```python
from build123d import *

# Parameters (mm, degrees)
SKETCH8_W           = 114.3
SKETCH8_H           = 38.1
BOSS_EXTRUDE3_DEPTH = 19.05


with BuildPart() as part:
    # Sketch8 → Boss-Extrude3 (new body)
    with BuildSketch(Plane.XY):
        with BuildLine():
            Line((-257.351483657, 282.913503235), (-304.976483657, 282.913503235))
            Line((-304.976483657, 282.913503235), (-304.976483657, 244.813503235))
            ThreePointArc((-304.976483657, 244.813503235), (-301.801483657, 241.638503235), (-304.976483657, 238.463503235))
            Line((-304.976483657, 238.463503235), (-324.026483657, 238.463503235))
            Line((-324.026483657, 238.463503235), (-324.026483657, 219.413503235))
            Line((-324.026483657, 219.413503235), (-304.976483657, 219.413503235))
            ThreePointArc((-304.976483657, 219.413503235), (-301.801483657, 216.238503235), (-304.976483657, 213.063503235))
            Line((-304.976483657, 213.063503235), (-304.976483657, 111.463503235))
            ThreePointArc((-304.976483657, 111.463503235), (-301.801483657, 108.288503235), (-304.976483657, 105.113503235))
            Line((-304.976483657, 105.113503235), (-324.026483657, 105.113503235))
            Line((-324.026483657, 105.113503235), (-324.026483657, 86.063503235))
            Line((-324.026483657, 86.063503235), (-304.976483657, 86.063503235))
            ThreePointArc((-304.976483657, 86.063503235), (-301.801483657, 82.888503235), (-304.976483657, 79.713503235))
            Line((-304.976483657, 79.713503235), (-304.976483657, -21.886496765))
            ThreePointArc((-304.976483657, -21.886496765), (-301.801483657, -25.061496765), (-304.976483657, -28.236496765))
            Line((-304.976483657, -28.236496765), (-324.026483657, -28.236496765))
            Line((-324.026483657, -28.236496765), (-324.026483657, -47.286496765))
            Line((-324.026483657, -47.286496765), (-304.976483657, -47.286496765))
            ThreePointArc((-304.976483657, -47.286496765), (-301.801483657, -50.461496765), (-304.976483657, -53.636496765))
            Line((-304.976483657, -53.636496765), (-304.976483657, -155.236496765))
            ThreePointArc((-304.976483657, -155.236496765), (-301.801483657, -158.411496765), (-304.976483657, -161.586496765))
            Line((-304.976483657, -161.586496765), (-324.026483657, -161.586496765))
            Line((-324.026483657, -161.586496765), (-324.026483657, -180.636496765))
            Line((-324.026483657, -180.636496765), (-304.976483657, -180.636496765))
            ThreePointArc((-304.976483657, -180.636496765), (-301.801483657, -183.811496765), (-304.976483657, -186.986496765))
            Line((-304.976483657, -186.986496765), (-304.976483657, -266.361496765))
            Line((-304.976483657, -266.361496765), (304.623516343, -266.361496765))
            Line((304.623516343, -266.361496765), (304.623516343, -186.986496765))
            ThreePointArc((304.623516343, -186.986496765), (301.448516343, -183.811496765), (304.623516343, -180.636496765))
            Line((304.623516343, -180.636496765), (323.673516343, -180.636496765))
            Line((323.673516343, -180.636496765), (323.673516343, -161.586496765))
            Line((323.673516343, -161.586496765), (304.623516343, -161.586496765))
            ThreePointArc((304.623516343, -161.586496765), (301.448516343, -158.411496765), (304.623516343, -155.236496765))
            Line((304.623516343, -155.236496765), (304.623516343, -53.636496765))
            ThreePointArc((304.623516343, -53.636496765), (301.448516343, -50.461496765), (304.623516343, -47.286496765))
            Line((304.623516343, -47.286496765), (323.673516343, -47.286496765))
            Line((323.673516343, -47.286496765), (323.673516343, -28.236496765))
            Line((323.673516343, -28.236496765), (304.623516343, -28.236496765))
            ThreePointArc((304.623516343, -28.236496765), (301.448516343, -25.061496765), (304.623516343, -21.886496765))
            Line((304.623516343, -21.886496765), (304.623516343, 79.713503235))
            ThreePointArc((304.623516343, 79.713503235), (301.448516343, 82.888503235), (304.623516343, 86.063503235))
            Line((304.623516343, 86.063503235), (323.673516343, 86.063503235))
            Line((323.673516343, 86.063503235), (323.673516343, 105.113503235))
            Line((323.673516343, 105.113503235), (304.623516343, 105.113503235))
            ThreePointArc((304.623516343, 105.113503235), (301.448516343, 108.288503235), (304.623516343, 111.463503235))
            Line((304.623516343, 111.463503235), (304.623516343, 213.063503235))
            ThreePointArc((304.623516343, 213.063503235), (301.448516343, 216.238503235), (304.623516343, 219.413503235))
            Line((304.623516343, 219.413503235), (323.673516343, 219.413503235))
            Line((323.673516343, 219.413503235), (323.673516343, 238.463503235))
            Line((323.673516343, 238.463503235), (304.623516343, 238.463503235))
            ThreePointArc((304.623516343, 238.463503235), (301.448516343, 241.638503235), (304.623516343, 244.813503235))
            Line((304.623516343, 244.813503235), (304.623516343, 282.913503235))
            Line((304.623516343, 282.913503235), (276.048516343, 282.913503235))
            Line((276.048516343, 282.913503235), (276.048516343, 247.988503235))
            Line((276.048516343, 247.988503235), (161.748516343, 247.988503235))
            Line((161.748516343, 247.988503235), (161.748516343, 282.913503235))
            Line((161.748516343, 282.913503235), (66.498516343, 282.913503235))
            Line((66.498516343, 282.913503235), (66.498516343, 247.988503235))
            Line((66.498516343, 247.988503235), (-47.801483657, 247.988503235))
            Line((-47.801483657, 247.988503235), (-47.801483657, 282.913503235))
            Line((-47.801483657, 282.913503235), (-143.051483657, 282.913503235))
            Line((-143.051483657, 282.913503235), (-143.051483657, 247.988503235))
            Line((-143.051483657, 247.988503235), (-257.351483657, 247.988503235))
            Line((-257.351483657, 247.988503235), (-257.351483657, 282.913503235))
        make_face()
        with Locations((-200.201483657, -133.011496765)):
            Rectangle(SKETCH8_W, SKETCH8_H, mode=Mode.SUBTRACT)
        with Locations((-200.201483657, 0.338503235)):
            Rectangle(SKETCH8_W, SKETCH8_H, mode=Mode.SUBTRACT)
        with Locations((9.348516343, -133.011496765)):
            Rectangle(SKETCH8_W, SKETCH8_H, mode=Mode.SUBTRACT)
        with Locations((218.898516343, -133.011496765)):
            Rectangle(SKETCH8_W, SKETCH8_H, mode=Mode.SUBTRACT)
        with Locations((9.348516343, 0.338503235)):
            Rectangle(SKETCH8_W, SKETCH8_H, mode=Mode.SUBTRACT)
        with Locations((218.898516343, 0.338503235)):
            Rectangle(SKETCH8_W, SKETCH8_H, mode=Mode.SUBTRACT)
        with Locations((-200.201483657, 133.688503235)):
            Rectangle(SKETCH8_W, SKETCH8_H, mode=Mode.SUBTRACT)
        with Locations((9.348516343, 133.688503235)):
            Rectangle(SKETCH8_W, SKETCH8_H, mode=Mode.SUBTRACT)
        with Locations((218.898516343, 133.688503235)):
            Rectangle(SKETCH8_W, SKETCH8_H, mode=Mode.SUBTRACT)
    extrude(amount=BOSS_EXTRUDE3_DEPTH)


solid = part.part
```
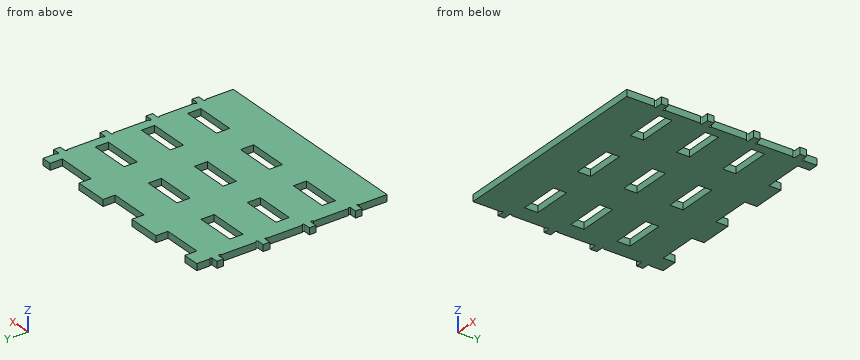
Design review of the part built by this model. Coordinates are the model's own, in mm. Coordinates: 2 decimals unless noted, no trailing zeros. Order: outer loops, then holes, each group sorted by start corner. A loop starts at its lowest first (then second) coordinate and runs counter-clockwise, first axis right, second up.
1) Take a section at B-B, the plane y = -121.5. Give the boundary of the cut face in (x, z), and give its area (3 significant figures).
2) Take a section at C-C, the plane z = 4.75. State how many separate pieces and enclosed holes the cut face has, and give its area (3 significant figures).
3) Wall thickness on line 1 along Y through (x, z) = (5, 16); line 2 along X through (y, z) = (125, 12); line 3 along X through (y, z) = (170.5, 8.75): over which ranges is each line inside the solid? List them lowest first.
4) Clearance check with flat-ended pins moving along their axes: pin 1 (1 mm diameter, centred on y = -82, z = 11, fed in from -X); pin 2 (9.5 mm diameter, centred on x = -310, z = 13, fed in from -Y); pin 3 (5.5 mm diameter, centred on y = 260.5, z = 12, fed in from +X). State where each tip first meets the part, or that it passes through.
5) Take a section at A-A, the plane x = 196.5. Give the boundary of the cut face in (y, z).
Returned:
1. outline: (-304.98, 0) - (-257.35, 0) - (-257.35, 19.05) - (-304.98, 19.05) - close; (-143.05, 0) - (-47.8, 0) - (-47.8, 19.05) - (-143.05, 19.05) - close; (66.5, 0) - (161.75, 0) - (161.75, 19.05) - (66.5, 19.05) - close; (276.05, 0) - (304.62, 0) - (304.62, 19.05) - (276.05, 19.05) - close
1. area: 5,080 mm2
2. separate pieces: 1
2. enclosed holes: 9
2. area: 286,000 mm2
3. line 1: y = -266.36 to -152.06, -113.96 to -18.71, 19.39 to 114.64, 152.74 to 247.99
3. line 2: x = -304.98 to -257.35, -143.05 to -47.8, 66.5 to 161.75, 276.05 to 304.62
3. line 3: x = -304.98 to 304.62
4. pin 1: stops at x = -304.98
4. pin 2: stops at y = -180.64
4. pin 3: stops at x = 304.62
5. outline: (-266.36, 0) - (-152.06, 0) - (-152.06, 19.05) - (-266.36, 19.05) - close; (-113.96, 0) - (-18.71, 0) - (-18.71, 19.05) - (-113.96, 19.05) - close; (19.39, 0) - (114.64, 0) - (114.64, 19.05) - (19.39, 19.05) - close; (152.74, 0) - (247.99, 0) - (247.99, 19.05) - (152.74, 19.05) - close
